Source: CAD feature listing. Evaluate the final solid. Frame: model axes, mm. A direction names the side the tool comes from. Coordinates: 2 decimals unless noted, no trailing zeros. Loops run counter-clockwise (first coordinate to the right, second up) from the corner with the lowest first, then second, coordinate; pieces in that order, holes last.
Solid Edge part; units mm, degrees
sketch "Sketch1" plane through (0, 0, 0) normal (0, 0, 1) x (1, 0, 0)
  line L0 (-4.25, -2.75) -> (4.25, -2.75)
  line L1 (4.25, -2.75) -> (4.25, 2.75)
  line L2 (4.25, 2.75) -> (-4.25, 2.75)
  line L3 (-4.25, 2.75) -> (-4.25, -2.75)
  dimension "D1" = 4.25
  dimension "D2" = 4.25
extrude "Protrusion1" add sketch "Sketch1" along normal blind 1.2
sketch "Sketch2" plane through (0, 0, 1.2) normal (0, 0, 1) x (1, 0, 0)
  line L0 (-3.85, -0.9) -> (-2.55, -0.9)
  line L1 (-2.55, -0.9) -> (-2.55, 0.4)
  line L2 (-2.55, 0.4) -> (-3.85, 0.4)
  line L3 (-3.85, 0.4) -> (-3.85, -0.9)
  line L4 (-0.25, -0.9) -> (-0.25, 0.4)
  line L5 (-0.25, 0.4) -> (-1.55, 0.4)
  line L6 (-1.55, 0.4) -> (-1.55, -0.9)
  line L7 (-1.55, -0.9) -> (-0.25, -0.9)
  line L8 (0.0122, 0.6689) -> (1.6122, 0.6689)
  line L9 (1.6122, 0.6689) -> (1.6122, 0.8689)
  line L10 (1.6122, 0.8689) -> (0.0122, 0.8689)
  line L11 (0.0122, 0.8689) -> (0.0122, 0.6689)
  line L12 (2.0787, 0.6689) -> (3.6787, 0.6689)
  line L13 (3.6787, 0.6689) -> (3.6787, 0.8689)
  line L14 (3.6787, 0.8689) -> (2.0787, 0.8689)
  line L15 (2.0787, 0.8689) -> (2.0787, 0.6689)
  dimension "D1" = 2.55
  dimension "D2" = 3.85
extrude "boutons" add sketch "Sketch2" along normal blind 0.8212
Q1. Section C-C, the plane y = -0.05. Return the cut outline in (x, z), plus the area to 3 significant figures.
Q2. Section B-B, the plane z = 1.55. Return the cut outline in (x, y).
Q3. Section A-A, the plane x = 3.5. Return the cut outline in (y, z).
Q4. Section D-D, the plane x = -3.25. Return the cut outline in (y, z).
Q5. Line query: line 1 along X through (y, z) = (-0.8, 1.65); line 2 along Z through (x, y) = (-3.5, -1.45); line 3 along Y through (x, z) = (-3.25, 1.5). Output: solid intervals per line, ascending.
Q6. Access query for faces 5 (the flat face through (0.8, 0.869, 1.6)), 6 (the flat face through (0, 0, 0)), 7 (the flat face through (2.9, 0.669, 1.6)), 8 (the flat face through (-1, 0, 2.021)), 9 (the flat face through (-3.85, -0.2, 1.6)). Directions: +Z, -Z, +X, -X, +Y, -Y. A direction counts if a zero-diameter tool reaches every point of the face in a straight line with its end or side. Return the directions, or none.
Q7. Draft query along X for faces 1 (the flat face through (-3, 0, 2.021)), 2 (the flat face through (-1.55, -0.2, 1.6)), 3 (the flat face through (-0.25, -0.3, 1.6)), 4 (the flat face through (-4.25, 0, 1)). Return one class per face: +X half, -X half, draft (parallel to the pull), parting line (faces both ways), or undercut.
Derived:
1. outline: (-4.25, 0) - (4.25, 0) - (4.25, 1.2) - (-0.25, 1.2) - (-0.25, 2.02) - (-1.55, 2.02) - (-1.55, 1.2) - (-2.55, 1.2) - (-2.55, 2.02) - (-3.85, 2.02) - (-3.85, 1.2) - (-4.25, 1.2) - close
1. area: 12.3 mm2
2. outline: (-3.85, -0.9) - (-2.55, -0.9) - (-2.55, 0.4) - (-3.85, 0.4) - close; (-1.55, -0.9) - (-0.25, -0.9) - (-0.25, 0.4) - (-1.55, 0.4) - close; (0.01, 0.67) - (1.61, 0.67) - (1.61, 0.87) - (0.01, 0.87) - close; (2.08, 0.67) - (3.68, 0.67) - (3.68, 0.87) - (2.08, 0.87) - close
3. outline: (-2.75, 0) - (2.75, 0) - (2.75, 1.2) - (0.87, 1.2) - (0.87, 2.02) - (0.67, 2.02) - (0.67, 1.2) - (-2.75, 1.2) - close
4. outline: (-2.75, 0) - (2.75, 0) - (2.75, 1.2) - (0.4, 1.2) - (0.4, 2.02) - (-0.9, 2.02) - (-0.9, 1.2) - (-2.75, 1.2) - close
5. line 1: x = -3.85 to -2.55, -1.55 to -0.25
5. line 2: z = 0 to 1.2
5. line 3: y = -0.9 to 0.4
6. face 5: +Z, +X, -X, +Y
6. face 6: -Z, +X, -X, +Y, -Y
6. face 7: +Z, +X, -X, -Y
6. face 8: +Z, +X, -X, +Y, -Y
6. face 9: +Z, -X, +Y, -Y
7. face 1: draft
7. face 2: undercut
7. face 3: +X half
7. face 4: -X half
